Check sheet for the drawn part. Datum: minimum x, y, z corner. Units: mm. A direction names the side the tool comes from. Round coordinates to 2 decimals unless told otherwise and drop trailing zeros. Loops run counter-clockwise (first coordinate to the right, second up) from the corner with the lowest first, then second, coordinate; pieces in that order, holes last. Notation, with made-up numbers: (-20.75, 4.5) -> (9.25, 4.5) arc R12 cw to (9.25, 8.5) -> close; hole circle Ø11 at (82, -31.5). An arc over 180 degrees is marked (long way). Return JSON: item names as keys, results as strings.
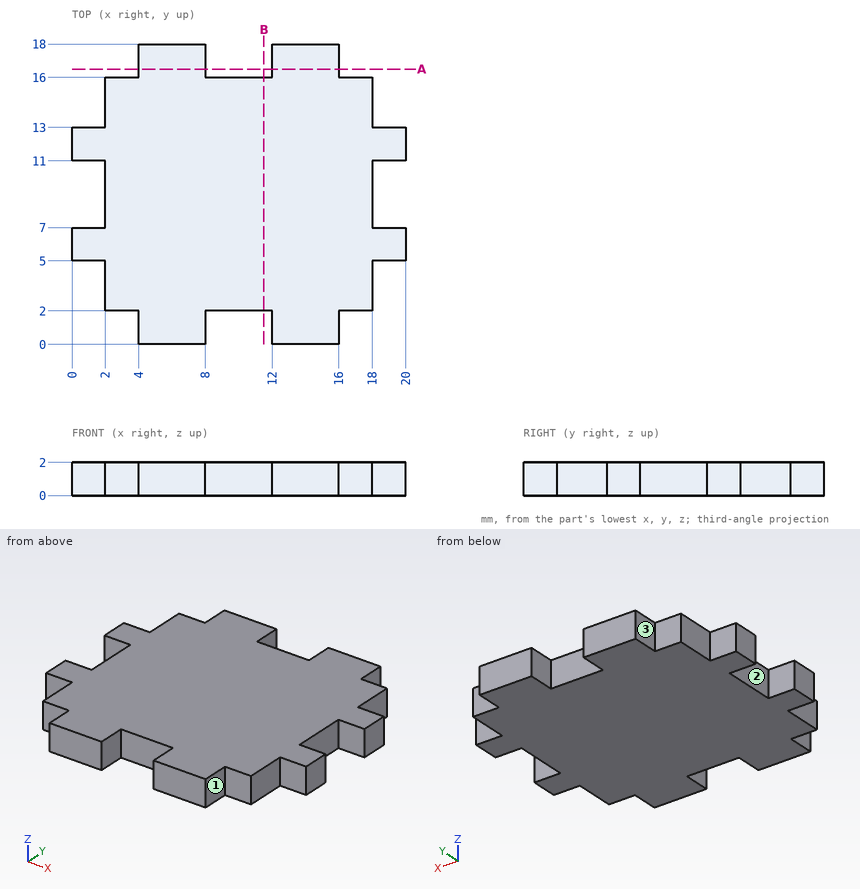
Q1. Material ranges on line 1 (Y direction, x = 1.75, z = 0.8); line 2 (X direction, y = 1.25, z = 1.2); line 3 (Y direction, x = 2.5, z = 1.2), recorded low to high.
Results list:
{"line 1": "5 to 7, 11 to 13", "line 2": "4 to 8, 12 to 16", "line 3": "2 to 16"}
Q2. Tool access check on the marked faces 1, 2 and 3. Record the directions out of +Z, -Z, +X, -X, +Y, -Y that give a thin tool (end or side, any length) a straight path to the whole face; none if there is none.
Results list:
{"face 1": "+Z, -Z, +X, -Y", "face 2": "+Z, -Z, -X", "face 3": "+Z, -Z, -X, +Y"}
Q3. Section check A-A (y = 16.5). Record the boundary of the cut face in (x, z), then the cut area to 3 significant figures.
Results list:
{"outline": "(4, 0) -> (8, 0) -> (8, 2) -> (4, 2) -> close; (12, 0) -> (16, 0) -> (16, 2) -> (12, 2) -> close", "area": "16.0 mm^2"}
Q4. Go/stop test with flat-tipped pins: pin 1 (1 mm diameter, centred on y = 3, z = 1, fed in from -X); pin 2 (0.6 mm diameter, centred on x = 17.5, z = 1.5, fed in from -Y); pin 3 (0.6 mm diameter, centred on x = 18.5, z = 0.5, fed in from -Y). Record where each tip stops, or that it passes through.
Results list:
{"pin 1": "x = 2", "pin 2": "y = 2", "pin 3": "y = 5"}
Q5. Section check B-B (x = 11.5). Record the boundary of the cut face in (y, z).
Results list:
{"outline": "(2, 0) -> (16, 0) -> (16, 2) -> (2, 2) -> close"}
